The figure shows three views and two pictorial views of one solid part (mm, origin at its lowest corner). Answer the questions. A direction names the side the tool comes from. Round coordinates to 2 decimals unless told otherwise and drop trailing zeros. Loops run counter-clockwise (first coordinate to the right, second up) from the corner with the lowest first, then second, coordinate; pieces in that order, holes last. Notation, with made-up numbers: (-19, 1.25) -> (22, 1.25) arc R21 ccw to (22, 6.25) -> close; hole circle Ø5 at (-3.5, 47.5). An arc over 180 degrees is marked (long way). Put each result on its own line as item: value.
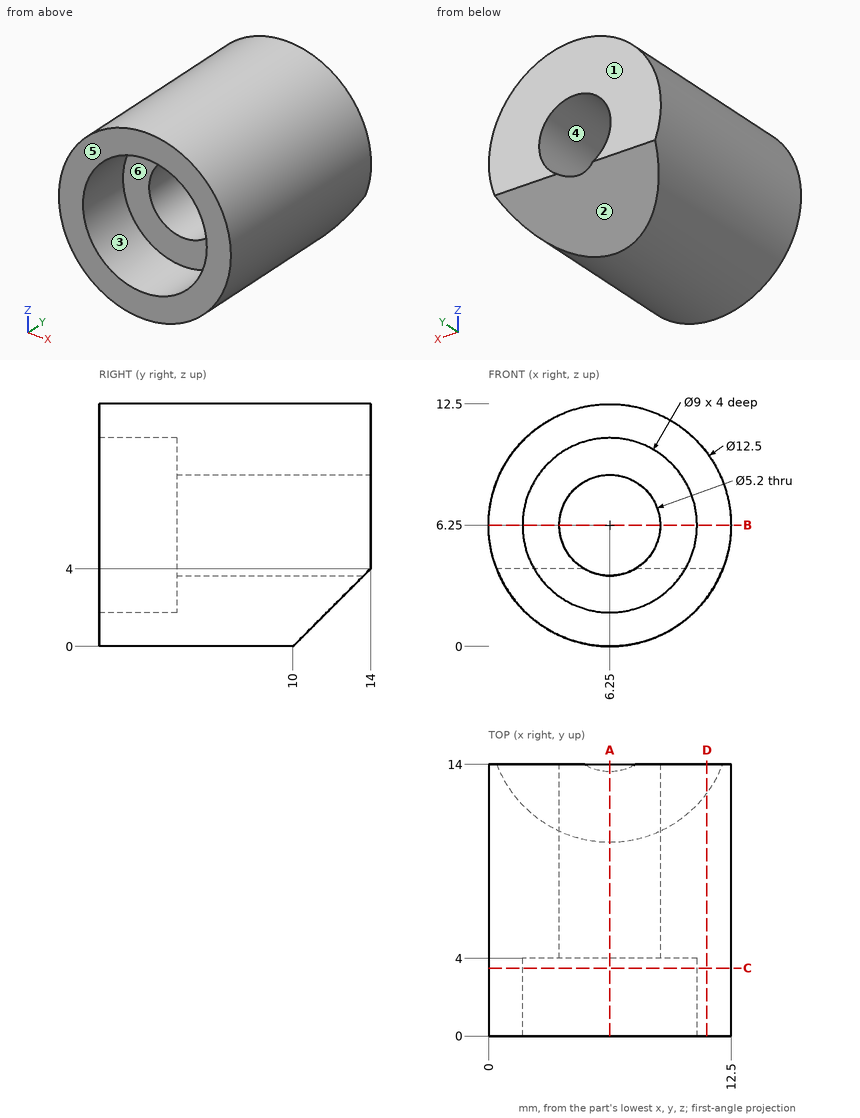
Item 1: The part is cut by section C-C (y = 3.5). Determine the outline of the cut face in (x, z), then the cut area to 3 significant figures.
Derived:
outline: circle Ø12.5 at (6.25, 6.25); hole circle Ø9 at (6.25, 6.25)
area: 59.1 mm^2
Item 2: The part is cut by section D-D (x = 11.25). Determine the outline of the cut face in (y, z), then the cut area to 3 significant figures.
Derived:
outline: (0, 2.5) -> (12.5, 2.5) -> (14, 4) -> (14, 10) -> (0, 10) -> close
area: 104 mm^2
Item 3: For a pull along Z with two mould halves and no side action, classify the marked faces 1, 2, 3 and 4 as pulls with the +Z half, pulls with the -Z half, needs draft (parallel to the pull), parting line crosses it, or undercut.
Derived:
face 1: needs draft
face 2: pulls with the -Z half
face 3: undercut
face 4: undercut
Item 4: Find the intervals of material crossed by line 1 along Z through (x, y) = (6.25, 3.05); line 2 along X through (y, z) = (10, 6.25); line 3 along Y through (x, z) = (9.75, 8.25), in increasing order.
Derived:
line 1: z = 0 to 1.75, 10.75 to 12.5
line 2: x = 0 to 3.65, 8.85 to 12.5
line 3: y = 4 to 14
Item 5: The part is cut by section A-A (x = 6.25). Determine the outline of the cut face in (y, z).
Derived:
outline: (0, 0) -> (10, 0) -> (13.65, 3.65) -> (4, 3.65) -> (4, 1.75) -> (0, 1.75) -> close; (0, 10.75) -> (4, 10.75) -> (4, 8.85) -> (14, 8.85) -> (14, 12.5) -> (0, 12.5) -> close
Item 6: Flat-ended cylindrical pins translate along their axes: pin 1 Ø1.5 at (y, z) = (8, 9.5) entering from +X; pin 2 Ø2 at (x, y) = (2, 6) entering from -Z; pin 3 Ø4.5 at (x, z) = (6.25, 6.25) entering from -Y; pin 4 Ø6 at (y, z) = (8.5, 9.5) entering from -X (3 decimals). Find the tip coordinate at first contact, or state that the pin passes through.
Derived:
pin 1: stops at x = 11.98
pin 2: stops at z = 0.91
pin 3: passes through
pin 4: stops at x = 0.005
Item 7: The part is cut by section B-B (z = 6.25). Determine the outline of the cut face in (x, y).
Derived:
outline: (0, 0) -> (1.75, 0) -> (1.75, 4) -> (3.65, 4) -> (3.65, 14) -> (0, 14) -> close; (8.85, 4) -> (10.75, 4) -> (10.75, 0) -> (12.5, 0) -> (12.5, 14) -> (8.85, 14) -> close
Item 8: Which of the six approach directions +Z, -Z, +X, -X, +Y, -Y give full straight-line access (tool end or side, diameter ignored) to the marked faces 5 and 6?
Derived:
face 5: +Z, -Z, +X, -X, -Y
face 6: -Y
